Source: CAD feature listing. Evaluate the final solid. Frame: model axes, mm. Round coordinates to 2 decimals unless told otherwise and drop trailing zeros. Order: outer loops, then holes, each group sorted by start corner. A loop starts at its lowest first (then second) coordinate and runs counter-clockwise, first axis right, second up. Notation, with made-up numbers: (65, -20.75) - (82, -20.75) arc R28 ccw to (82, 11.25) - close; hole circle Ø9 at (15, 58.25). An arc over 180 degrees is marked (long way). Use one line per item in the form item = value. Start each with the question number.
Q1. Draft query along Y for faces 1 (the cylindrical face through (31, 9.76, 0.16)), 2 (the flat face through (0, -6, -13.5)), 3 (the cylindrical face through (-0.54, -2.44, 0.19)). Return one class per face: released by +Y, released by -Y, zero draft, split by the parting line, or undercut.
Q2. Ray query, line 1 (Y direction, x = 0, z = -5.75); line 2 (Y direction, x = -1.5, z = 12); line 3 (Y direction, x = 29.5, z = 4). Return the intervals inside material, ascending. Write a range as [from, to].
Q3. Pin query (flat end, axial travel): pin 1 Ø5 at (y, z) = (5.5, -10) entering from +X; pin 2 Ø3 at (y, z) = (-10.5, -9) entering from +X; pin 3 Ø3 at (x, y) = (0, 0) entering from +Z; pin 4 Ø1.5 at (y, z) = (4, 7) entering from -X. Return the tip coordinate at first contact, or that it passes through.
Q4. Cut plane C-C, the plane z = 7.25. Return the cut outline in (x, y).
Q5. Cut plane A-A, the plane y = 0. Return the cut outline in (x, z), and give its area (3 significant figures).
from build123d import *

# Parameters (mm, degrees)
SKETCH1_R           = 32.5
BOSS_EXTRUDE1_DEPTH = 13.5
FILLET1_R           = 2
SKETCH2_R           = 2.5
CUT_EXTRUDE1_DEPTH  = 28


with BuildPart() as part:
    # Sketch1 → Boss-Extrude1 (new body, symmetric)
    with BuildSketch(Plane.XY):
        Circle(SKETCH1_R)
    extrude(amount=BOSS_EXTRUDE1_DEPTH, both=True)

    # Fillet1
    fillet1_edges = [part.edges().sort_by_distance(p)[0] for p in [
        (-32.5, 0, -13.5),
        (-32.5, 0, 13.5),
    ]]
    fillet(fillet1_edges, radius=FILLET1_R)

    # Sketch2 → Cut-Extrude1 (cut, through all)
    with BuildSketch(Plane.XY.offset(13.5)):
        Circle(SKETCH2_R)
    extrude(amount=-CUT_EXTRUDE1_DEPTH, mode=Mode.SUBTRACT)


solid = part.part
Completed:
q1.face_1 = split by the parting line
q1.face_2 = zero draft
q1.face_3 = undercut
q2.line_1 = [-32.5, -2.5], [2.5, 32.5]
q2.line_2 = [-32.4, -2], [2, 32.4]
q2.line_3 = [-13.64, 13.64]
q3.pin_1 = 32.36
q3.pin_2 = 31.23
q3.pin_3 = through
q3.pin_4 = -32.34
q4.outline = circle Ø65 at (0, 0); hole circle Ø5 at (0, 0)
q5.outline = (-32.5, -11.5) arc R2 ccw to (-30.5, -13.5) - (-2.5, -13.5) - (-2.5, 13.5) - (-30.5, 13.5) arc R2 ccw to (-32.5, 11.5) - close; (2.5, -13.5) - (30.5, -13.5) arc R2 ccw to (32.5, -11.5) - (32.5, 11.5) arc R2 ccw to (30.5, 13.5) - (2.5, 13.5) - close
q5.area = 1,620 mm2
